Work out the finished part from the listing and answer in its coordinate system (mm). Face numbers are marked on the shaded views. Round coordinates to 2 decimals unless told otherwise and drop trailing zeros. Write each loop counter-clockwise with the first axis right and the second up, starting at its lowest first coordinate (ties: lowest second). Pieces come first, ordered by that corner, then holes.
1. Straight lines are drawn through the part: probe 1 along Y at (x, z) = (-2, -2.25); probe 2 along X at (y, z) = (1.25, 3); probe 3 along Y at (x, z) = (-1, -2.5). For each, find the intervals that lie inside material, in ascending order.
2. Determine the mould class of the marked faces 1, 2, 3 and 4 for opening direction X: pulls with the +X half, pulls with the -X half, needs draft (parallel to the pull), parting line crosses it, or undercut.
3. Find section A-A (z = 3.25). Write down the section's boundary in (x, y).
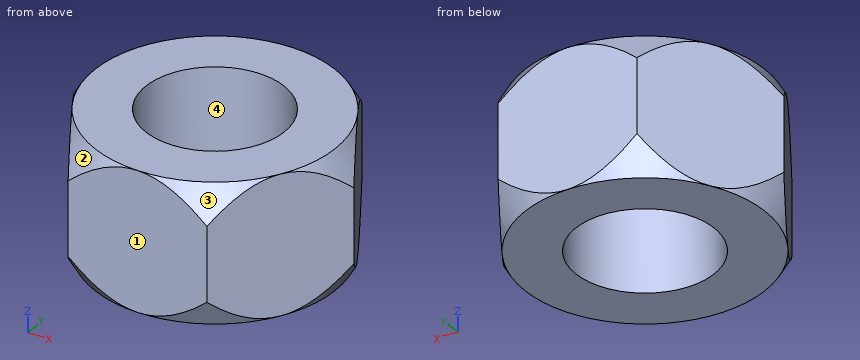
```python
from build123d import *

# Parameters (mm, degrees)
BOSS_EXTRUDE1_DEPTH     = 4
SKETCH2_OUTSIDE_W       = 31.764
SKETCH2_OUTSIDE_H       = 29.62
SKETCH2_OUTSIDE_R       = 6.92820323
CUT_EXTRUDE1_DEPTH      = 8
CUT_EXTRUDE1_DRAFT      = -30
MIRROR1_COPY_1_SKETCH_W = 31.764
MIRROR1_COPY_1_SKETCH_H = 29.62
MIRROR1_COPY_1_SKETCH_R = 6.92820323
MIRROR1_COPY_1_DEPTH    = 8
MIRROR1_COPY_1_DRAFT    = -30
SKETCH3_R               = 4
CUT_EXTRUDE2_DEPTH      = 8


with BuildPart() as part:
    # Sketch1 → Boss-Extrude1 (new, symmetric)
    with BuildSketch(Plane.XY):
        Polygon((8, 0), (4, 6.92820323), (-4, 6.92820323), (-8, 0), (-4, -6.92820323), (4, -6.92820323), align=None)
    extrude(amount=BOSS_EXTRUDE1_DEPTH, both=True)


with BuildPart() as cut_extrude1_tool:
    # Sketch2 outside → Cut-Extrude1 (with draft: the straight prism first)
    with BuildSketch(Plane.XY.offset(4)):
        Rectangle(SKETCH2_OUTSIDE_W, SKETCH2_OUTSIDE_H)
        Circle(SKETCH2_OUTSIDE_R, mode=Mode.SUBTRACT)
    extrude(amount=-CUT_EXTRUDE1_DEPTH)
    # Cut-Extrude1: the draft: its side faces are tilted about the plane it starts from
    cut_extrude1_sides = [cut_extrude1_tool.faces().sort_by_distance(p)[0] for p in [
        (0, -14.81, 0),
        (15.882, 0, 0),
        (0, 14.81, 0),
        (-15.882, 0, 0),
        (-6.92820323, 0, 0),
    ]]
    draft(cut_extrude1_sides, Plane.XY.offset(4), CUT_EXTRUDE1_DRAFT)


with BuildPart() as part_1:
    add(part.part)

    # Cut-Extrude1: cut by cut_extrude1_tool
    add(cut_extrude1_tool.part, mode=Mode.SUBTRACT)


with BuildPart() as mirror1_copy_1_tool:
    # Mirror1 copy 1 sketch → Mirror1 copy 1 (with draft: the straight prism first)
    with BuildSketch(Plane(origin=(0, 0, -4), x_dir=(1, 0, 0), z_dir=(0, 0, -1))):
        Rectangle(MIRROR1_COPY_1_SKETCH_W, MIRROR1_COPY_1_SKETCH_H)
        Circle(MIRROR1_COPY_1_SKETCH_R, mode=Mode.SUBTRACT)
    extrude(amount=-MIRROR1_COPY_1_DEPTH)
    # Mirror1 copy 1: the draft: its side faces are tilted about the plane it starts from
    mirror1_copy_1_sides = [mirror1_copy_1_tool.faces().sort_by_distance(p)[0] for p in [
        (0, -14.81, 0),
        (15.882, 0, 0),
        (0, 14.81, 0),
        (-15.882, 0, 0),
        (-6.92820323, 0, 0),
    ]]
    draft(mirror1_copy_1_sides, Plane(origin=(0, 0, -4), x_dir=(1, 0, 0), z_dir=(0, 0, -1)), MIRROR1_COPY_1_DRAFT)


with BuildPart() as part_2:
    add(part_1.part)

    # Mirror1 copy 1: cut by mirror1_copy_1_tool
    add(mirror1_copy_1_tool.part, mode=Mode.SUBTRACT)

    # Sketch3 → Cut-Extrude2 (cut)
    with BuildSketch(Plane.XY.offset(4)):
        Circle(SKETCH3_R)
    extrude(amount=-CUT_EXTRUDE2_DEPTH, mode=Mode.SUBTRACT)


solid = part_2.part
```
Worked answers:
1. probe 1: y = -6.93 to -3.46, 3.46 to 6.93
1. probe 2: x = -7.28 to -3.8, 3.8 to 7.28
1. probe 3: y = -6.93 to -3.87, 3.87 to 6.93
2. face 1: needs draft
2. face 2: pulls with the -X half
2. face 3: pulls with the +X half
2. face 4: undercut
3. outline: (-7.24, -1.31) - (-4.76, -5.62) arc R7.36 ccw to (-2.49, -6.93) - (2.49, -6.93) arc R7.36 ccw to (4.76, -5.62) - (7.24, -1.31) arc R7.36 ccw to (7.24, 1.31) - (4.76, 5.62) arc R7.36 ccw to (2.49, 6.93) - (-2.49, 6.93) arc R7.36 ccw to (-4.76, 5.62) - (-7.24, 1.31) arc R7.36 ccw to start; hole circle Ø8 at (0, 0)
